The model under review builds one solid part; all positions refer to its coordinate system, in mm. Face numbers are marked on the shaded views. A direction names the side the tool comes from. Give positions to 0.01 mm unless a question says otherwise; leave off trailing zeros. Order: outer loops, then holes, each group sorted by start corner. A loop starts at its lowest first (then second) coordinate and runs counter-clockwise, first axis right, second up. Notation, with made-up numbers: (-29.5, 64) -> (-13.5, 64) arc R10 ccw to (-13.5, 75) -> close; hole circle Ø10 at (11, 6). An arc over 180 degrees is marked (long way). Use one line per item in the form item = value.
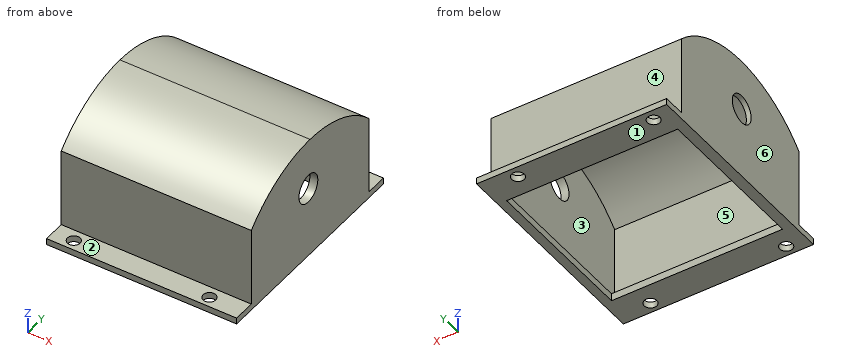
```python
from build123d import *

# Parameters (mm, degrees)
EXTRUDE051_DEPTH                          = 56
SKETCH049_R                               = 2
EXTRUDE049_DEPTH                          = 15
SKETCH048_R                               = 4.5
EXTRUDE048_DEPTH                          = 100
SKETCH046_AS_DRAWN_W                      = 50
SKETCH046_AS_DRAWN_H                      = 54
EXTRUDE046_DEPTH                          = 24
EXTRUDE046_ONTO_SKETCH046_PITCH_ANGLE     = 0.457086
EXTRUDE046_ONTO_SKETCH046_PLACEMENT_ANGLE = 90
EXTRUDE045_DEPTH                          = 60


with BuildPart() as obj1:
    # Sketch050 (on Face1 of Cut026) → Extrude051 (new body)
    with BuildSketch(Plane(origin=(-35.5, 0, 0), x_dir=(0, -1, 0), z_dir=(-1, 0, 0))):
        with BuildLine():
            Line((24.067108, 62.828769), (24.067108, 39.546181))
            Line((24.067108, 39.546181), (78.067085, 39.546181))
            Line((78.067085, 62.712322), (78.067085, 39.546181))
            ThreePointArc((78.067085, 62.712322), (51.091637, 74.150565), (24.067108, 62.828769))
        make_face()
    extrude(amount=EXTRUDE051_DEPTH)


with BuildPart() as obj1_1:
    # Extrude051 placement: moved
    add(obj1.part.moved(Location((57.5, 0, 0))))


with BuildPart() as weapon_cover_screw_holes:
    # Sketch049 (on Face6 of Cut025) → Extrude049 (new body, symmetric)
    with BuildSketch(Plane.XY.offset(39.2)):
        with Locations((-29.074951, -82.714325)):
            Circle(SKETCH049_R)
        with Locations((13.75458, -82.714325)):
            Circle(SKETCH049_R)
        with Locations((-29.074951, -19.516283)):
            Circle(SKETCH049_R)
        with Locations((13.75458, -19.516283)):
            Circle(SKETCH049_R)
    extrude(amount=EXTRUDE049_DEPTH, both=True)


with BuildPart() as axis_hole_lid:
    # Sketch048 (on Face3 of Cut024) → Extrude048 (new body, symmetric)
    with BuildSketch(Plane.YZ.offset(24.5)):
        with Locations((-51.79294, 59.926255)):
            Circle(SKETCH048_R)
    extrude(amount=EXTRUDE048_DEPTH, both=True)


with BuildPart() as obj2:
    # Sketch046 as drawn → Extrude046 (new)
    with BuildSketch(Plane.XY):
        with Locations((-9, -1)):
            Rectangle(SKETCH046_AS_DRAWN_W, SKETCH046_AS_DRAWN_H)
    extrude(amount=EXTRUDE046_DEPTH)


with BuildPart() as obj2_1:
    # Extrude046 onto Sketch046 pitch: moved
    add(obj2.part.rotate(Axis((0, 0, 0), (0, 1, 0)), EXTRUDE046_ONTO_SKETCH046_PITCH_ANGLE))


with BuildPart() as obj2_2:
    # Extrude046 onto Sketch046 placement: moved
    add(obj2_1.part.moved(Location((-5.5, -69.445946, 37.254054))).rotate(Axis((-5.5, -69.445946, 37.254054), (0, 0, 1)), EXTRUDE046_ONTO_SKETCH046_PLACEMENT_ANGLE))


with BuildPart() as obj2_3:
    # Extrude046 placement: moved
    add(obj2_2.part.moved(Location((-0.75, 27.25, -1))))


with BuildPart() as weapon_gear_cover:
    # Sketch045 → Extrude045 (new body)
    with BuildSketch(Plane.YZ):
        with BuildLine():
            Line((-86, 37.2), (-86, 39.2))
            Line((-86, 39.2), (-79, 39.2))
            Line((-79, 39.2), (-79, 64.2))
            ThreePointArc((-51, 76.097301), (-66.211392, 72.999631), (-79, 64.2))
            ThreePointArc((-23, 64.2), (-35.788608, 72.999631), (-51, 76.097301))
            Line((-23, 39.2), (-23, 64.2))
            Line((-16, 39.2), (-23, 39.2))
            Line((-16, 37.2), (-16, 39.2))
            Line((-16, 37.2), (-51, 37.2))
            Line((-86, 37.2), (-51, 37.2))
        make_face()
    extrude(amount=EXTRUDE045_DEPTH)


with BuildPart() as weapon_gear_cover_1:
    # Extrude045 placement: moved
    add(weapon_gear_cover.part.moved(Location((-35.5, 0, 0))))

    # Cut024: cut obj2
    add(obj2_3.part, mode=Mode.SUBTRACT)

    # Cut025: cut Axis Hole Lid
    add(axis_hole_lid.part, mode=Mode.SUBTRACT)

    # Cut026: cut Weapon Cover Screw Holes
    add(weapon_cover_screw_holes.part, mode=Mode.SUBTRACT)

    # Cut028: cut obj1
    add(obj1_1.part, mode=Mode.SUBTRACT)


solid = weapon_gear_cover_1.part
```
1. The part is to be moulded in two halves that separate along X. For the marked faces 4, 5 and 6, say which applies: +X half, -X half, draft (parallel to the pull), parting line (faces both ways), or undercut.
Values:
face_4 = draft
face_5 = undercut
face_6 = -X half
2. Tool access review of the marked faces 1, 2 and 3: name each direction out of +Z, -Z, +X, -X, +Y, -Y from which nothing blocks a thin tool from reaching the whole face with its end or side.
Values:
face_1 = -Z, +X, -X, +Y, -Y
face_2 = +Z, +X, -X, -Y
face_3 = none
3. Add section B-B on z = 57.5. Give the boundary of the cut face in (x, y), then the cut area to 3 significant figures.
Values:
outline = (-35.5, -79) -> (24.5, -79) -> (24.5, -55.58) -> (22, -55.58) -> (22, -78.07) -> (-34, -78.07) -> (-34, -55.58) -> (-35.5, -55.58) -> close; (-35.5, -48) -> (-34, -48) -> (-34, -24.07) -> (22, -24.07) -> (22, -48) -> (24.5, -48) -> (24.5, -23) -> (-35.5, -23) -> close
area = 306 mm^2
4. Add section A-A on z = 46. Give the boundary of the cut face in (x, y).
Values:
outline = (-35.5, -79) -> (24.5, -79) -> (24.5, -23) -> (-35.5, -23) -> close; hole (-34, -78.07) -> (22, -78.07) -> (22, -24.07) -> (-34, -24.07) -> close
5. Add section D-D on y = -75. Give the boundary of the cut face in (x, z), then the cut area to 3 significant figures.
Values:
outline = (-35.5, 37.2) -> (-32.25, 37.2) -> (-32.25, 39.55) -> (-34, 39.55) -> (-34, 65.54) -> (22, 65.54) -> (22, 39.55) -> (21.75, 39.55) -> (21.75, 37.2) -> (24.5, 37.2) -> (24.5, 67.81) -> (-35.5, 67.81) -> close
area = 254 mm^2
6. Add section C-C on x = 7.5. Give the boundary of the cut face in (y, z).
Values:
outline = (-86, 37.2) -> (-76.19, 37.2) -> (-76.17, 39.55) -> (-78.07, 39.55) -> (-78.07, 62.71) arc R37.72 cw to (-24.07, 62.83) -> (-24.07, 39.55) -> (-26.17, 39.55) -> (-26.19, 37.2) -> (-16, 37.2) -> (-16, 39.2) -> (-23, 39.2) -> (-23, 64.2) arc R38.9 ccw to (-79, 64.2) -> (-79, 39.2) -> (-86, 39.2) -> close
7. For pin 1 Ø8 at (x, y) = (-14.5, -29) entering from +Z; pin 2 Ø5.5 at (y, z) = (-51.79, 59.93) entering from -X; pin 3 Ø7.5 at (x, z) = (7, 54.5) entering from +Y; pin 4 Ø2 at (x, y) = (5.5, -20.5) entering from +Z, all flat-tipped, find the tip position at first contact; note any pin that passes through.
Values:
pin_1 = 71.68
pin_2 = through
pin_3 = -23
pin_4 = 39.2
8. For L1, parallel to Y at x = -32.5, z = 51.5; L2, parallel to X at y = -45.5, z = 66; L3, parallel to Y at x = -17.5, z = 69, list the stretches that pass through material, from the lowest coordinate up.
Values:
L1 = -79 to -78.07, -24.07 to -23
L2 = -35.5 to -34, 22 to 24.5
L3 = -73.4 to -70.04, -31.98 to -28.6
